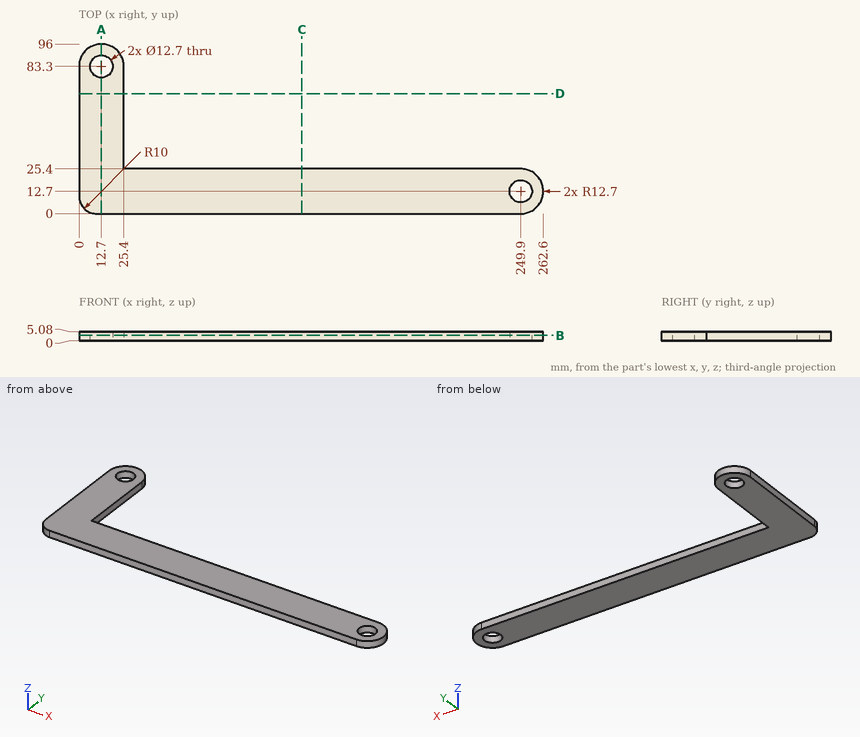
Verification items for this drawing (mm, ordinates from the low corner). Coordinates: 2 decimals unless noted, no trailing zeros. Write each loop counter-clockwise with the first axis right and the second up, starting at its lowest first coordinate (ties: lowest second). Pieces come first, ordered by that corner, then holes. Notation, with made-up numbers: (49.5, 81) -> (84.5, 81) arc R14 ccw to (84.5, 86) -> close; hole circle Ø7 at (72, 17). An arc over 180 degrees is marked (long way). One line per item, written item: value. Start each with the question number.
Q1. Cross-section at A-A on x = 12.7. Enter the section's corners in (y, z), and give its area (3 significant figures).
Q2. Go/stop test with flat-tipped pins: P1, Ø1, axis at y = 81, z = 2.5, coming from the +X side; P2, Ø2.5, axis at x = 116, z = 3, coming from the +Y side. Record where each tip stops, or that it passes through.
Q3. Cross-section at B-B on z = 3.05. Enter the section's corners in (x, y), and give its area (3 significant figures).
Q4. Thickness scan on L1, parallel to X at y = 82.5, z = 0.8; L2, parallel to Y at x = 139.5, z = 1.9. Record the ranges inside material, lowest first. Write a range as from..to.
Q5. Cross-section at C-C on x = 126. Enter the section's corners in (y, z).
Checked values:
1. outline: (0, 0) -> (76.95, 0) -> (76.95, 5.08) -> (0, 5.08) -> close; (89.65, 0) -> (96, 0) -> (96, 5.08) -> (89.65, 5.08) -> close
1. area: 423 mm²
2. P1: stops at x = 25.4
2. P2: stops at y = 25.4
3. outline: (0, 10) arc R10 ccw to (10, 0) -> (249.9, 0) arc R12.7 ccw to (249.9, 25.4) -> (25.4, 25.4) -> (25.4, 83.3) arc R12.7 ccw to (0, 83.3) -> close; hole circle Ø12.7 at (12.7, 83.3); hole circle Ø12.7 at (249.9, 12.7)
3. area: 8,050 mm²
4. L1: x = 0..6.4, 19..25.4
4. L2: y = 0..25.4
5. outline: (0, 0) -> (25.4, 0) -> (25.4, 5.08) -> (0, 5.08) -> close
